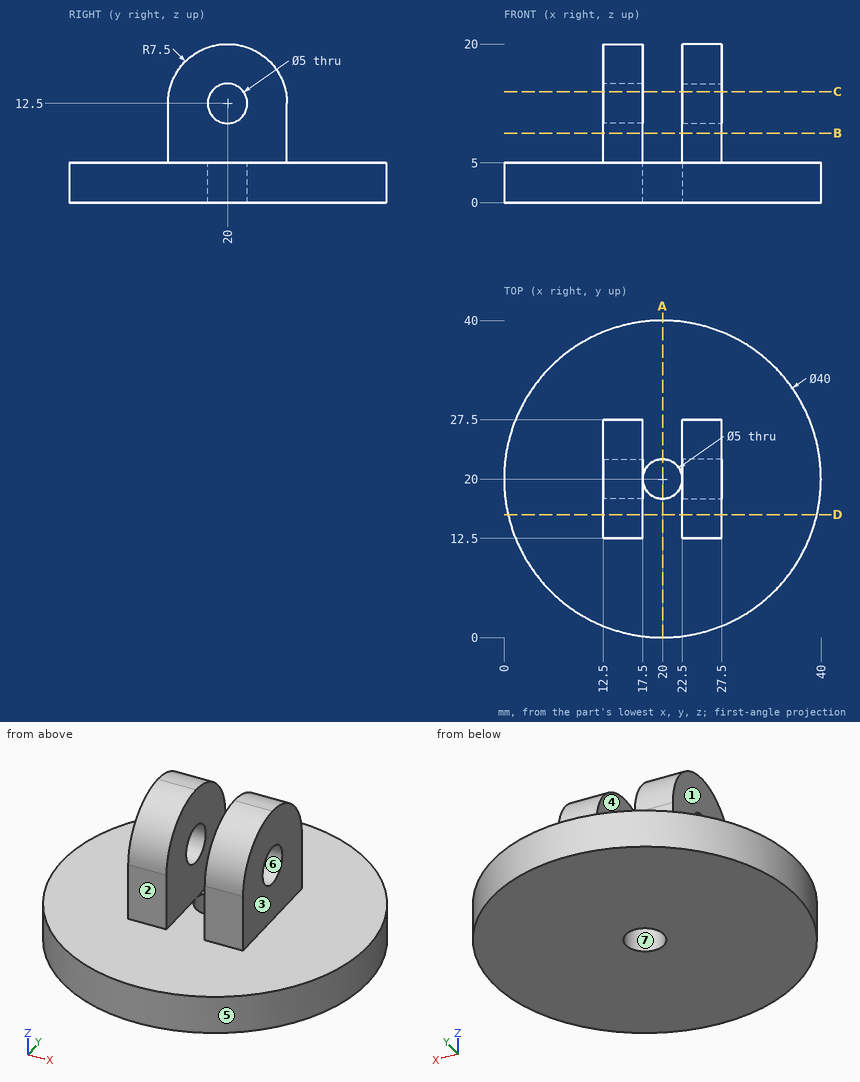
Geometry: see drawing. Coordinates: mm, zero at the bounding-box minimum. A direction names the side the tool comes from. Give positions to 0.01 mm unless a question says otherwise; leave off trailing zeros. Loops run counter-clockwise (first coordinate to the right, second up) from the corner with the lowest first, then second, coordinate; pieces in that order, holes last. Notation, with made-up numbers: (56.5, 53.25) - (64.5, 53.25) arc R16 ccw to (64.5, 65.25) - close; hole circle Ø4 at (0.25, 56). An arc over 180 degrees is marked (long way). Use CSV: the item, a comma, the result in double quotes.
1) Mould query, pull axis X, two halves, no side actions, for the marked faces 5, 6 and 7. Classes: +X half, -X half, draft (parallel to the pull), parting line (faces both ways), or undercut.
Worked out:
face 5,"parting line"
face 6,"draft"
face 7,"undercut"
2) Cut plane C-C (z = 14). Output: boundary loops of the cut face in (x, y), and give its area (3 significant figures).
Worked out:
outline,"(12.5, 12.65) - (17.5, 12.65) - (17.5, 18) - (12.5, 18) - close; (12.5, 22) - (17.5, 22) - (17.5, 27.35) - (12.5, 27.35) - close; (22.5, 12.65) - (27.5, 12.65) - (27.5, 18) - (22.5, 18) - close; (22.5, 22) - (27.5, 22) - (27.5, 27.35) - (22.5, 27.35) - close"
area,"107 mm^2"
3) Cut plane B-B (z = 8.75). Output: boundary loops of the cut face in (x, y).
Worked out:
outline,"(12.5, 12.5) - (17.5, 12.5) - (17.5, 27.5) - (12.5, 27.5) - close; (22.5, 12.5) - (27.5, 12.5) - (27.5, 27.5) - (22.5, 27.5) - close"
4) Line query: line 1 (X direction, y = 13.5, z = 13.5); line 2 (Z direction, x = 11, y = 30); line 3 (Y direction, x = 20, z = 2.8). Output: solid intervals per line, ascending.
Worked out:
line 1,"x = 12.5 to 17.5, 22.5 to 27.5"
line 2,"z = 0 to 5"
line 3,"y = 0 to 17.5, 22.5 to 40"
5) Pin query (flat end, axial travel): P1, Ø5, axis at x = 20.5, y = 25.5, coming from the +Z side; P2, Ø10, axis at x = 19, y = 27.5, coming from the -Z side; P3, Ø4, axis at x = 20, y = 20, coming from the +Z side; P4, Ø4, axis at x = 15, y = 10, coming from the +Z side. Return the tip coordinate at first contact, or that it passes through.
Worked out:
P1,"stops at z = 18.84"
P2,"stops at z = 0"
P3,"passes through"
P4,"stops at z = 5"
6) Cut plane D-D (y = 15.5). Output: boundary loops of the cut face in (x, z), and give its area (3 significant figures).
Worked out:
outline,"(0.51, 0) - (39.49, 0) - (39.49, 5) - (27.5, 5) - (27.5, 18.5) - (22.5, 18.5) - (22.5, 5) - (17.5, 5) - (17.5, 18.5) - (12.5, 18.5) - (12.5, 5) - (0.51, 5) - close"
area,"330 mm^2"
7) Set-up query: the marked faces 1, 2, 3 and 4. Return all of +Z, -Z, +X, -X, +Y, -Y with unobstructed straight access to the full face (end or side cutting, diameter ignored); none if empty.
Worked out:
face 1,"+Z, -X, +Y, -Y"
face 2,"+Z, +X, -X, -Y"
face 3,"+Z, +X, +Y, -Y"
face 4,"+Z, +Y, -Y"
8) Cut plane A-A (x = 20). Output: boundary loops of the cut face in (y, z), and give its area (3 significant figures).
Worked out:
outline,"(0, 0) - (17.5, 0) - (17.5, 5) - (0, 5) - close; (22.5, 0) - (40, 0) - (40, 5) - (22.5, 5) - close"
area,"175 mm^2"
